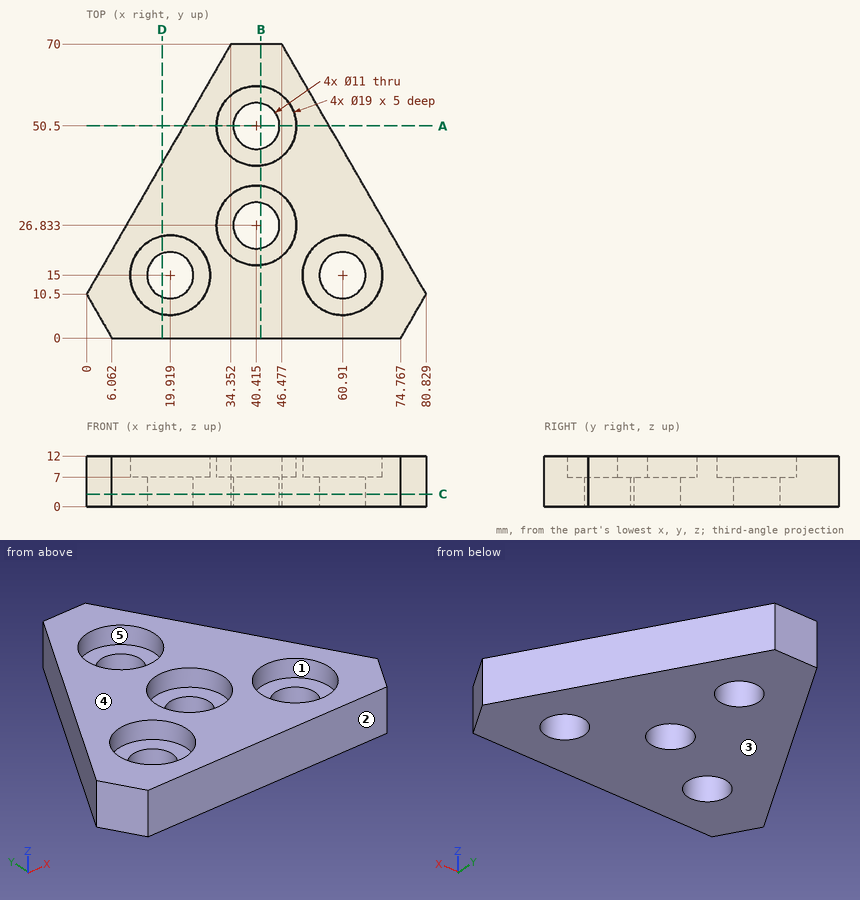
Input: dimensioned drawing with shaded views. Units: mm. Origin: part minimum x, y, z. A direction names the side the tool comes from. Round coordinates to 2 decimals unless told otherwise and drop trailing zeros. Loops run counter-clockwise (first coordinate to the right, second up) from the corner with the lowest first, then second, coordinate; pieces in that order, holes last.
1) Set-up query: the marked faces 4 and 5. Return all of +Z, -Z, +X, -X, +Y, -Y with unobstructed straight access to the full face (end or side cutting, diameter ignored); none if empty.
Ans:
face 4: +Z, +X, -X, +Y, -Y
face 5: +Z
2) Section query C-C on z = 3. Return the cut outline in (x, y) (1 decimal).
Ans:
outline: (0, 10.5) - (6.1, 0) - (74.8, 0) - (80.8, 10.5) - (46.5, 70) - (34.4, 70) - close; hole circle Ø11 at (19.9, 15); hole circle Ø11 at (40.4, 26.8); hole circle Ø11 at (40.4, 50.5); hole circle Ø11 at (60.9, 15)
3) Material intervals for line 1 (X direction, y = 12.5, z = 7.75) (1 decimal); line 2 (Y direction, x = 47.5, z = 8.5) (1 decimal); line 3 (X direction, y = 11, z = 8) (1 decimal), sorted ascending.
Ans:
line 1: x = 1.2 to 10.8, 29.1 to 51.7, 70.1 to 79.7
line 2: y = 0 to 20.5, 33.2 to 44.2, 56.8 to 68.2
line 3: x = 0.3 to 11.3, 28.5 to 52.3, 69.5 to 80.5
4) Section query B-B on x = 41.5. Return the cut outline in (y, z) (1 decimal), plus the area to 3 significant figures.
Ans:
outline: (0, 0) - (21.4, 0) - (21.4, 7) - (17.4, 7) - (17.4, 12) - (0, 12) - close; (32.2, 0) - (45.1, 0) - (45.1, 7) - (41.1, 7) - (41.1, 12) - (36.3, 12) - (36.3, 7) - (32.2, 7) - close; (55.9, 0) - (70, 0) - (70, 12) - (59.9, 12) - (59.9, 7) - (55.9, 7) - close
area: 500 mm2
5) Pin query (flat end, axial travel): pin 1 (2 mm diameter, centred on y = 32.5, z = 5.5, fed in from -X) (1 decimal); pin 2 (3 mm diameter, centred on x = 48.5, z = 6.5, fed in from +Y) (1 decimal); pin 3 (11.5 mm diameter, centred on x = 19.92, y = 15, fed in from +Z). Return the tip coordinate at first contact, or that it passes through.
Ans:
pin 1: stops at x = 12.1
pin 2: stops at y = 69.1
pin 3: stops at z = 7
6) Pull-direction query (Y, two-part tool) for the marked faces 1, 2 and 3; classes: released by +Y, released by -Y, zero draft, split by the parting line, or undercut.
Ans:
face 1: undercut
face 2: released by -Y
face 3: zero draft
7) Section query D-D on x = 18. Return the cut outline in (y, z) (1 decimal), plus the area to 3 significant figures.
Ans:
outline: (0, 0) - (9.8, 0) - (9.8, 7) - (5.7, 7) - (5.7, 12) - (0, 12) - close; (20.2, 0) - (41.7, 0) - (41.7, 12) - (24.3, 12) - (24.3, 7) - (20.2, 7) - close
area: 335 mm2
8) Section query A-A on y = 50.5. Return the cut outline in (x, z) (1 decimal).
Ans:
outline: (23.1, 0) - (34.9, 0) - (34.9, 7) - (30.9, 7) - (30.9, 12) - (23.1, 12) - close; (45.9, 0) - (57.7, 0) - (57.7, 12) - (49.9, 12) - (49.9, 7) - (45.9, 7) - close
